Can you work these out from the model? Positions are in its coordinate system, mm. A direction names the side the tool comes from. Coordinates: 2 decimals unless noted, no trailing zeros. Write each loop counter-clockwise with the first axis right and the second up, starting at its lowest first coordinate (ties: lowest second). Pieces come first, ordered by that corner, then holes. Notation, with made-up numbers: (42.5, 44) - (80.5, 44) arc R21 cw to (80.5, 73) - close; hole circle Ø6 at (73, -6.75). An arc over 180 degrees is marked (long way). Use one line per item in the form item = value. Start each with the question number.
(1) Thinking about a two-plate mould opening in Y: for faces 4 (the face through (-145.635, 12, 5)), 5 (the face through (-135.635, -18, 5)), which applies, pulls with the +Y half, pulls with the -Y half, needs draft (parallel to the pull), parting line crosses it, or undercut?
(2) On a 3-axis mill with a long thin cutter (end or side, diameter ignored), from which of +Z, -Z, +X, -X, +Y, -Y can I reach the whole of each face in a straight line? I mean faces 1 (the face through (-135.635, 2, 5)), 2 (the face through (131.165, -18, 5)), 3 (the face through (-4, -7, 0)). Say none if no direction works.
(3) If we section it at C-C on x = 121: Please give me the cut outline in (y, z).
(4) If we section it at B-B on y = 3: Please give me the cut outline in (x, z), then the cut area to 3 significant figures.
(5) For pin 1 Ø5 at (x, z) = (-140, 7) entering from -Y; pin 2 Ø5 at (x, z) = (57, 4.5) entering from -Y; pin 3 Ø5 at (y, z) = (1.5, 6) entering from +X, each with a flat end and sliding along its axis, tell me the tip position at first contact or that it passes through.
(6) If I drill on probe 1 along X at (y, z) = (17, 7.5); probe 2 along Y at (x, z) = (126, 5.75); probe 3 along Y at (x, z) = (10.5, 1.5), over which ranges is the centre line in solid material (lowest first)? Write a range as from..to.
```python
from build123d import *

# Parameters (mm, degrees)
F0_W     = 10
F0_H     = 10
F1_DEPTH = 10


# Not quite as in the source:
# - a feature names something its author has since deleted; it is built from what else it names


with BuildPart() as f1:
    # F0 (on Top) → F1 (new body)
    with BuildSketch(Plane.XY):
        Polygon((131.1653250098, 36.9413525529), (-135.6346749902, 36.9413525529), (-135.6346749902, 26.9413525529), (-135.6346749902, 16.9413525529), (-135.6346749902, 6.9413525529), (-135.6346749902, -3.0586474471), (-135.6346749902, -13.0586474471), (-135.6346749902, -23.0586474471), (-135.6346749902, -33.0586474471), (131.1653250098, -33.0586474471), (131.1653250098, -23.0586474471), (131.1653250098, -13.0586474471), (131.1653250098, -3.0586474471), (131.1653250098, 6.9413525529), (131.1653250098, 16.9413525529), (131.1653250098, 26.9413525529), align=None)
        with Locations((-140.6346749902, 31.9413525529)):
            Rectangle(F0_W, F0_H)
        with Locations((-140.6346749902, 11.9413525529)):
            Rectangle(F0_W, F0_H)
        with Locations((-140.6346749902, -8.0586474471)):
            Rectangle(F0_W, F0_H)
        with Locations((-140.6346749902, -28.0586474471)):
            Rectangle(F0_W, F0_H)
        with Locations((136.1653250098, 31.9413525529)):
            Rectangle(F0_W, F0_H)
        with Locations((136.1653250098, 11.9413525529)):
            Rectangle(F0_W, F0_H)
        with Locations((136.1653250098, -8.0586474471)):
            Rectangle(F0_W, F0_H)
        with Locations((136.1653250098, -28.0586474471)):
            Rectangle(F0_W, F0_H)
        Polygon((-135.6346749902, -33.0586474471), (-145.6346749902, -33.0586474471), (131.1653250098, -52.3612973773), (131.1653250098, -43.0586474471), (131.1653250098, -33.0586474471), align=None)
        Polygon((131.1653250098, -43.0586474471), (131.1653250098, -52.3612973773), (141.1653250098, -53.0586474471), (141.1653250098, -43.0586474471), align=None)
    extrude(amount=F1_DEPTH)


solid = f1.part
```
Reported:
q1.face_4 = needs draft
q1.face_5 = undercut
q2.face_1 = +Z, -Z, -X
q2.face_2 = +Z, -Z, +X
q2.face_3 = -Z, +X, -X, +Y, -Y
q3.outline = (-51.65, 0) - (36.94, 0) - (36.94, 10) - (-51.65, 10) - close
q4.outline = (-135.63, 0) - (131.17, 0) - (131.17, 10) - (-135.63, 10) - close
q4.area = 2,670 mm2
q5.pin_1 = -33.63
q5.pin_2 = -47.36
q5.pin_3 = 131.17
q6.probe_1 = -135.63..131.17
q6.probe_2 = -52..36.94
q6.probe_3 = -43.95..36.94
